The listing builds one solid part. Answer for the finished solid, in the listing's coordinates (mm). A direction names the side the tool comes from. Coordinates: 2 decimals unless noted, no trailing zeros. Order: outer loops, then holes, each group sorted by start corner. A loop starts at its lowest first (then second) coordinate and runs counter-clockwise, first axis right, second up. Notation, with made-up numbers: (48, 1.25) -> (90, 1.25) arc R17 ccw to (90, 22.25) -> close; hole circle Ø7 at (71, -33). An arc over 180 degrees is marked (long way). Return JSON: item names as keys, results as strings.
```python
from build123d import *

# Parameters (mm, degrees)
RESSALTO_EXTRUS_O1_DEPTH = 20
CORTE_EXTRUS_O1_DEPTH    = 54.150729064
ESBO_O3_R                = 2.25
CORTE_EXTRUS_O2_DEPTH    = 56.398555938
ESBO_O3_3_R              = 2.25
CUT_EXTRUDE1_DEPTH       = 4


with BuildPart() as part:
    # Esboço1 → Ressalto-extrusão1 (new body)
    with BuildSketch(Plane.XY):
        Polygon((0, 0), (0, 5), (13, 5), (13, 50), (20, 50), (20, 0), align=None)
    extrude(amount=RESSALTO_EXTRUS_O1_DEPTH)

    # Esboço2 → Corte-extrusão1 (cut, through all)
    with BuildSketch(Plane(origin=(0, 5, 0), x_dir=(1, 0, 0), z_dir=(0, 1, 0))):
        with BuildLine():
            Line((8.64, -3.75), (8.64, -16.25))
            ThreePointArc((8.64, -16.25), (6.39, -18.5), (4.14, -16.25))
            Line((4.14, -16.25), (4.14, -3.75))
            ThreePointArc((4.14, -3.75), (6.39, -1.5), (8.64, -3.75))
        make_face()
    extrude(amount=-CORTE_EXTRUS_O1_DEPTH, mode=Mode.SUBTRACT)

    # Esboço3 → Corte-extrusão2 (cut, through all)
    with BuildSketch(Plane.ZY.offset(-13)):
        with Locations((10, 35)):
            Circle(ESBO_O3_R)
        with Locations((10, 20)):
            Circle(ESBO_O3_R)
    extrude(amount=-CORTE_EXTRUS_O2_DEPTH, mode=Mode.SUBTRACT)

    # Esboço3<3> → Cut-Extrude1 (cut)
    # profile 1 of 2: a face of its own
    with BuildSketch(Plane.ZY.offset(-13)):
        Polygon((5.958548116, 20), (7.979274058, 16.5), (12.020725942, 16.5), (14.041451884, 20), (12.020725942, 23.5), (7.979274058, 23.5), align=None)
        with Locations((10, 20)):
            Circle(ESBO_O3_3_R, mode=Mode.SUBTRACT)
    # profile 2 of 2: a face of its own
    with BuildSketch(Plane.ZY.offset(-13)):
        Polygon((5.958548116, 35), (7.979274058, 31.5), (12.020725942, 31.5), (14.041451884, 35), (12.020725942, 38.5), (7.979274058, 38.5), align=None)
        with Locations((10, 35)):
            Circle(ESBO_O3_3_R, mode=Mode.SUBTRACT)
    extrude(amount=-CUT_EXTRUDE1_DEPTH, mode=Mode.SUBTRACT)


solid = part.part
```
Item 1: Flat-ended cylindrical pins translate along their axes: pin 1 (2.5 mm diameter, centred on y = 20, z = 10, fed in from +X); pin 2 (2 mm diameter, centred on y = 18.5, z = 8.5, fed in from -X); pin 3 (4 mm diameter, centred on x = 9, z = 11, fed in from +Y); pin 4 (10 mm diameter, centred on y = 30, z = 8, fed in from -X). Find the tip coordinate at first contact, or state that the pin passes through.
Answer list:
{"pin 1": "through", "pin 2": "x = 17", "pin 3": "y = 5", "pin 4": "x = 13"}
Item 2: Which of the six approach directions +Z, -Z, +X, -X, +Y, -Y give full straight-line access (tool end or side, diameter ignored) to faces 4 (the flat face through (15, 18.2, 13)), 5 (the cylindrical face through (18.48, 37.23, 9.71)), 6 (the cylindrical face through (6.3, 2.5, 1.5))?
Answer list:
{"face 4": "-X", "face 5": "+X, -X", "face 6": "+Y, -Y"}
Item 3: The part is cut by section A-A on z = 15. Determine the outline of the cut face in (x, y).
Answer list:
{"outline": "(0, 0) -> (4.14, 0) -> (4.14, 5) -> (0, 5) -> close; (8.64, 0) -> (20, 0) -> (20, 50) -> (13, 50) -> (13, 5) -> (8.64, 5) -> close"}
Item 4: Determine the mould class of faces 1 (the flat face through (15, 20, 20)), 2 (the flat face through (15, 38.5, 10)), 3 (the flat face through (3.5, 5, 9.9)) for opening direction Z: pulls with the +Z half, pulls with the -Z half, needs draft (parallel to the pull), parting line crosses it, or undercut.
Answer list:
{"face 1": "pulls with the +Z half", "face 2": "undercut", "face 3": "needs draft"}
Item 5: The part is cut by section C-C on z = 10. Determine the outline of the cut face in (x, y), plus the area to 4 significant figures.
Answer list:
{"outline": "(0, 0) -> (4.14, 0) -> (4.14, 5) -> (0, 5) -> close; (8.64, 0) -> (20, 0) -> (20, 17.75) -> (17, 17.75) -> (17, 16.5) -> (13, 16.5) -> (13, 5) -> (8.64, 5) -> close; (13, 23.5) -> (17, 23.5) -> (17, 22.25) -> (20, 22.25) -> (20, 32.75) -> (17, 32.75) -> (17, 31.5) -> (13, 31.5) -> close; (13, 38.5) -> (17, 38.5) -> (17, 37.25) -> (20, 37.25) -> (20, 50) -> (13, 50) -> close", "area": "309.5 mm2"}
Item 6: The part is cut by section D-D on y = 34.5. Determine the outline of the cut face in (x, z).
Answer list:
{"outline": "(13, 0) -> (20, 0) -> (20, 7.81) -> (17, 7.81) -> (17, 6.25) -> (13, 6.25) -> close; (13, 13.75) -> (17, 13.75) -> (17, 12.19) -> (20, 12.19) -> (20, 20) -> (13, 20) -> close"}
Item 7: Find the intervals of material crossed by probe 1 along Y at (x, z) = (18.5, 10); probe 2 along X at (y, z) = (11, 2.25); probe 3 along X at (y, z) = (37, 7.5), in increasing order.
Answer list:
{"probe 1": "0 to 17.75, 22.25 to 32.75, 37.25 to 50", "probe 2": "13 to 20", "probe 3": "17 to 20"}
Item 8: The part is cut by section B-B on x = 6.39. Determine the outline of the cut face in (y, z).
Answer list:
{"outline": "(0, 0) -> (5, 0) -> (5, 1.5) -> (0, 1.5) -> close; (0, 18.5) -> (5, 18.5) -> (5, 20) -> (0, 20) -> close"}
